Could you check a few things on this model? Use its own coordinates, in mm. A direction names the side the tool comes from. Give positions to 0.01 mm unless a question says otherwise; leave off trailing zeros. Order: outer loops, then holes, each group sorted by start corner. A loop starts at its lowest first (then second) coordinate and runs counter-clockwise, first axis right, second up. Notation, with made-up numbers: (27.25, 16) -> (56.25, 16) arc R13 ccw to (56.25, 35) -> close; hole circle Ø11 at (27, -9). An arc over 180 degrees is marked (long way). Write each question's results on one line, items separated by ' | '.
```python
from build123d import *

# Parameters (mm, degrees)
SKETCH1_W                    = 25.4
SKETCH1_H                    = 6.35
BOSS_EXTRUDE1_DEPTH          = 101.6
H_0_266_DIAMETER_HOLE1_D     = 6.7564
H_0_266_DIAMETER_HOLE1_DEPTH = 6.35
SKETCH4_W                    = 7.9375
SKETCH4_H                    = 25.4
CUT_EXTRUDE1_DEPTH           = 7.35


with BuildPart() as part:
    # Sketch1 → Boss-Extrude1 (new body)
    with BuildSketch(Plane(origin=(0, 0, 0), x_dir=(1, 0, 0), z_dir=(0, 1, 0))):
        with Locations((12.7, 3.175)):
            Rectangle(SKETCH1_W, SKETCH1_H)
    extrude(amount=BOSS_EXTRUDE1_DEPTH)

    # H (0.266) Diameter Hole1
    with Locations(Plane.XY):
        with Locations((12.7, 88.9), (12.7, 12.7)):
            Hole(H_0_266_DIAMETER_HOLE1_D / 2, depth=H_0_266_DIAMETER_HOLE1_DEPTH)

    # Sketch4 → Cut-Extrude1 (cut, through all)
    with BuildSketch(Plane(origin=(0, 0, -6.35), x_dir=(-1, 0, 0), z_dir=(0, 0, -1))):
        with Locations((-3.96875, 12.7)):
            Rectangle(SKETCH4_W, SKETCH4_H)
    extrude(amount=-CUT_EXTRUDE1_DEPTH, mode=Mode.SUBTRACT)


solid = part.part
```
Q1. I'm going to push flat-ended pins straight in: pin 1 Ø3 at (x, z) = (3, -4.5) entering from -Y; pin 2 Ø1.9 at (y, z) = (17.5, -4) entering from -X. Where does each tip first touch, or does it pass through?
Here are the results:
pin 1: stops at y = 25.4 | pin 2: stops at x = 7.94
Q2. For faces 5 (the flat face through (7.938, 13, -3)), 6 (the flat face through (13, 50, -6.35)), which set-ups out of +Z, -Z, +X, -X, +Y, -Y let a thin tool reach every point of the face, with its end or its side?
Here are the results:
face 5: +Z, -Z, -X, -Y | face 6: -Z, +X, -X, +Y, -Y
Q3. Suppose I cut it at C-C on z = -5.25. Please give me the cut outline in (x, y).
Here are the results:
outline: (0, 25.4) -> (7.94, 25.4) -> (7.94, 0) -> (25.4, 0) -> (25.4, 101.6) -> (0, 101.6) -> close; hole circle Ø6.76 at (12.7, 12.7); hole circle Ø6.76 at (12.7, 88.9)
Q4. Suppose I cut it at A-A on y = 88.9. Please give me the cut outline in (x, z), and give its area (3 significant figures).
Here are the results:
outline: (0, -6.35) -> (9.32, -6.35) -> (9.32, 0) -> (0, 0) -> close; (16.08, -6.35) -> (25.4, -6.35) -> (25.4, 0) -> (16.08, 0) -> close | area: 118 mm²
Q5. Suppose I cut it at B-B on x = 12.7. Please give me the cut outline in (y, z).
Here are the results:
outline: (0, -6.35) -> (9.32, -6.35) -> (9.32, 0) -> (0, 0) -> close; (16.08, -6.35) -> (85.52, -6.35) -> (85.52, 0) -> (16.08, 0) -> close; (92.28, -6.35) -> (101.6, -6.35) -> (101.6, 0) -> (92.28, 0) -> close
Q6. I need wall thicknesses on line 1 along Y through (x, z) = (12.7, -1.75); line 2 along Y through (x, z) = (12.25, -1.25); line 3 along Y through (x, z) = (7, -2.75). Which ranges of each line are inside material? Lowest first, please.
Here are the results:
line 1: y = 0 to 9.32, 16.08 to 85.52, 92.28 to 101.6 | line 2: y = 0 to 9.35, 16.05 to 85.55, 92.25 to 101.6 | line 3: y = 25.4 to 101.6
Q7. Suppose I cut it at D-D on y = 12.7. Please give me the cut outline in (x, z).
Here are the results:
outline: (7.94, -6.35) -> (9.32, -6.35) -> (9.32, 0) -> (7.94, 0) -> close; (16.08, -6.35) -> (25.4, -6.35) -> (25.4, 0) -> (16.08, 0) -> close
Q8. Thinking about a two-plate mould opening in Y: for faces 1 (the cylindrical face through (15.381, 10.644, -3.219)), 2 (the flat face through (0, 63, -3)), 3 (the flat face through (13, 101.6, -3)), 4 (the flat face through (4, 25.4, -3)), which applies, +Y half, -Y half, draft (parallel to the pull), parting line (faces both ways), or undercut?
Here are the results:
face 1: undercut | face 2: draft | face 3: +Y half | face 4: -Y half
